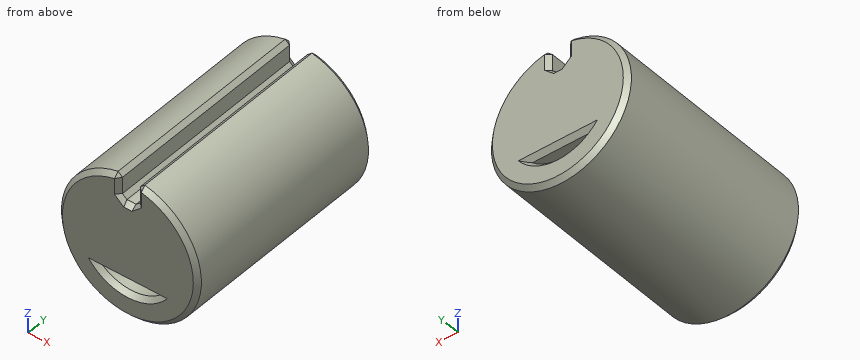
Autodesk Fusion 360 part; units mm, degrees
sketch "Sketch1" plane through (0, 0, 0) normal (0, 1, 0) x (1, 0, 0) in component "Coupler"
  circle A0 centre (0, 0) radius 3.9
  circle A1 centre (0, 0) radius 2.5
  line L0 (0, 0) -> (0, 1.9) construction
  line L1 (0, 1.9) -> (1.6248, 1.9)
  line L2 (0, 1.9) -> (-1.6248, 1.9)
  line L3 (0, 0) -> (0, -1.6667) construction
  line L4 (0, -1.6667) -> (0.5, -1.6667) construction
  line L5 (0, -1.6667) -> (-0.5, -1.6667) construction
  line L6 (0.5, -1.6667) -> (0.5, -3.8678)
  line L7 (-0.5, -1.6667) -> (-0.5, -3.8678)
  dimension "d6" = 7.8
  dimension "d7" = 5
  dimension "d8" = 1.9
  dimension "d9" = 1.6667
  dimension "d10" = 0.5
  dimension "d11" = 0.5
extrude "Extrude1" add sketch "Sketch1" along normal blind 12 contours A0 A1 L6 L7 | A1 L1 L2 picked at (-1.1759, -3.2181) picked at (-0.4526, -0.9659) in component "Coupler"
chamfer "Chamfer1" distance 0.25 angle 45 4 faces at (-0.1667, 12, -0.4502) (-0.1667, 0, -0.4502) (-0.5, 4, 2.9223) (0.5, 4, 2.9223) in component "Coupler"
component "Coupler" placed x (1, 0, 0) y (0, 1, 0) z (0, 0, 1) at (0, 0, 0)
equation "MotorShaftDiameter = 5 mm"
equation "MotorShaftKeyDiameter = 4.4 mm"
equation "CouplerDiameter = 7.8 mm"
equation "CouplerHeight = 12 mm"
equation "Gap = 1 mm"
equation "d6 = CouplerDiameter"
equation "d7 = MotorShaftDiameter"
equation "d8 = MotorShaftKeyDiameter - MotorShaftDiameter / 2"
equation "d9 = MotorShaftDiameter / 3"
equation "d10 = Gap / 2"
equation "d11 = d10"
equation "d12 = CouplerHeight"
Input: part model. Units: mm. Frame: model coordinates. Round coordinates to 2 decimals unless told otherwise and drop trailing zeros. Order: outer loops, then holes, each group sorted by start corner. A loop starts at its lowest first (then second) coordinate and runs counter-clockwise, first axis right, second up.
1. Cut plane A-A, the plane x = 0. Output: boundary loops of the cut face in (y, z), then the cut area to 4 significant figures.
The answers:
outline: (0, -3.65) - (0.25, -3.9) - (11.75, -3.9) - (12, -3.65) - (12, -2.75) - (11.75, -2.5) - (0.25, -2.5) - (0, -2.75) - close; (0, -1.65) - (0.25, -1.9) - (11.75, -1.9) - (12, -1.65) - (12, 2.25) - (11.75, 2.5) - (0.25, 2.5) - (0, 2.25) - close
area: 69.35 mm2
2. Material intervals for line 1 (Z direction, x = 1, y = 11.5); line 2 (Z direction, x = 1.25, y = 2.5); line 3 (X direction, y = 10.75, z = 3), sorted ascending.
The answers:
line 1: z = -3.77 to -2.29, -1.9 to 3.77
line 2: z = -3.69 to -2.17, -1.9 to 3.69
line 3: x = -2.49 to -0.5, 0.5 to 2.49
3. Pin query (flat end, axial travel): P1, Ø1, axis at x = -2, y = 11, coming from the -Z side. Return the tip coordinate at first contact, or that it passes through.
The answers:
P1: stops at z = -3.6
